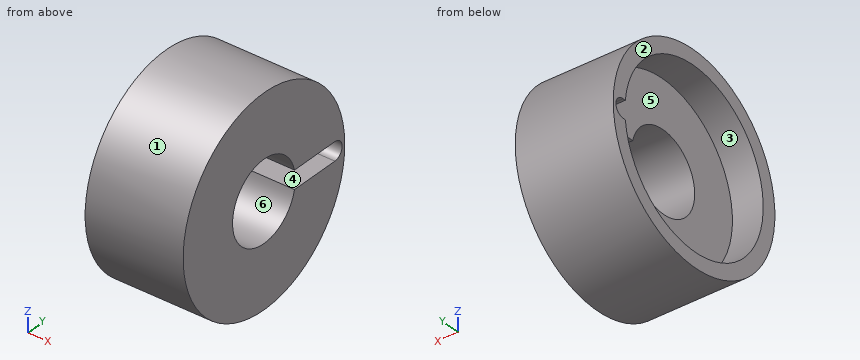
```python
from build123d import *

# Parameters (mm, degrees)
CUT_EXTRUDE1_REACH = 10.6


with BuildPart() as part:
    # Sketch3 → Revolve1 (revolve)
    with BuildSketch(Plane.XY):
        Polygon((253.385153788, -140.873704322), (253.385153788, -145.073704322), (259.285153788, -145.073704322), (259.285153788, -140.857236748), (259.285153788, -139.573704322), (250.685153788, -139.573704322), (250.685153788, -140.873704322), align=None)
    revolve(axis=Axis((227.370475166, -148.573704322, 0), (1, 0, 0)))

    # Sketch11 → Cut-Extrude1 (cut, up to next)
    with BuildSketch(Plane(origin=(259.285153788, 0, 0), x_dir=(0, 0, -1), z_dir=(1, 0, 0)), mode=Mode.PRIVATE) as cut_extrude1_sk1:
        with BuildLine():
            Line((-0.810006034, -140.673704322), (-0.810006034, -145.168724113))
            Line((-0.810006034, -145.168724113), (0.810006034, -145.168724113))
            Line((0.810006034, -145.168724113), (0.810006034, -140.673704322))
            ThreePointArc((0.810006034, -140.673704322), (0, -139.863698288), (-0.810006034, -140.673704322))
        make_face()
    cut_extrude1_tool1 = extrude(cut_extrude1_sk1.sketch, amount=-CUT_EXTRUDE1_REACH, mode=Mode.PRIVATE) & part.part
    add(cut_extrude1_tool1.solids().sort_by_distance((259.285154, -142.599941, 0))[0], mode=Mode.SUBTRACT)


solid = part.part
```
Could you check a few things on this model? Use its own coordinates, in mm. Face numbers are marked on the shaded views. A direction names the side the tool comes from. Round coordinates to 2 decimals unless told otherwise and drop trailing zeros. Loops run counter-clockwise (first coordinate to the right, second up) from the corner with the lowest first, then second, coordinate; pieces in that order, holes last. Notation, with made-up numbers: (69.5, 15) -> (87.5, 15) arc R33 ccw to (87.5, 44) -> close; hole circle Ø5 at (48, 62). An arc over 180 degrees is marked (long way). One line per question, with ' | ' between items.
(1) If we section it at D-D on z = 5.25: List the corners of the cut face in (x, y) for me, and give its area (3 significant figures).
Model answer:
outline: (250.69, -155.88) -> (259.29, -155.88) -> (259.29, -141.26) -> (250.69, -141.26) -> (250.69, -142.94) -> (253.39, -142.94) -> (253.39, -154.21) -> (250.69, -154.21) -> close | area: 95.3 mm^2
(2) For the marked faces 5 and 6, which set-ups out of +Z, -Z, +X, -X, +Y, -Y let a thin tool reach every point of the face, with its end or its side?
Model answer:
face 5: -X | face 6: +X, -X
(3) If I drill on probe 1 along X at (y, z) = (-155.25, 2); probe 2 along Z at (x, y) = (252, -153); probe 3 along Z at (x, y) = (252, -152.5), over which ranges is the centre line in solid material (lowest first)?
Model answer:
probe 1: x = 253.39 to 259.29 | probe 2: z = -7.84 to -6.3, 6.3 to 7.84 | probe 3: z = -8.1 to -6.62, 6.62 to 8.1
(4) If we section it at C-C on y = -153: List the corners of the cut face in (x, z) for me, and give its area (3 significant figures).
Model answer:
outline: (250.69, -7.84) -> (259.29, -7.84) -> (259.29, 7.84) -> (250.69, 7.84) -> (250.69, 6.3) -> (253.39, 6.3) -> (253.39, -6.3) -> (250.69, -6.3) -> close | area: 101 mm^2
(5) If we section it at A-A on z = 0: List the corners of the cut face in (x, y) for me, and give its area (3 significant figures).
Model answer:
outline: (250.69, -157.57) -> (259.29, -157.57) -> (259.29, -152.07) -> (253.39, -152.07) -> (253.39, -156.27) -> (250.69, -156.27) -> close; (250.69, -139.86) -> (259.29, -139.86) -> (259.29, -139.57) -> (250.69, -139.57) -> close | area: 38.5 mm^2
(6) Thinking about a two-plate mould opening in Z: for the marked faces 1, 2, 3 and 4, which applies, released by +Z, released by -Z, zero draft, split by the parting line, or undercut?
Model answer:
face 1: split by the parting line | face 2: zero draft | face 3: undercut | face 4: undercut
(7) For pin 1 Ø2 at (x, z) = (258, 7) entering from -Y; pin 2 Ø1.3 at (x, y) = (256, -142) entering from -Z; pin 3 Ø2 at (x, z) = (254, -2) entering from +Y; pin 4 Ø3 at (x, z) = (254, -1.5) entering from -Y, each with a flat end and sliding along its axis, tell me the tip position at first contact or that it passes through.
Model answer:
pin 1: stops at y = -155.28 | pin 2: stops at z = -6.78 | pin 3: stops at y = -139.63 | pin 4: stops at y = -157.57
(8) If we section it at B-B on y = -151: List the corners of the cut face in (x, z) for me, and give its area (3 significant figures).
Model answer:
outline: (250.69, -8.67) -> (259.29, -8.67) -> (259.29, -2.52) -> (253.39, -2.52) -> (253.39, -7.31) -> (250.69, -7.31) -> close; (250.69, 7.31) -> (253.39, 7.31) -> (253.39, 2.52) -> (259.29, 2.52) -> (259.29, 8.67) -> (250.69, 8.67) -> close | area: 79.8 mm^2
